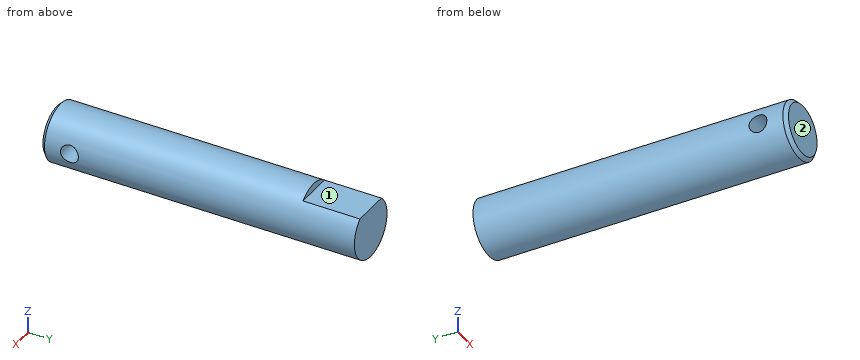
Autodesk Inventor part; units mm, degrees
ref_plane "Work Plane1" through (-4, 0, 0) normal (1, 0, 0) x (0, 1, 0)
ref_plane "XZ Plane" through (0, 0, 0) normal (0, 1, 0) x (-1, 0, 0)
ref_plane "XY Plane" through (0, 0, 0) normal (0, 0, 1) x (1, 0, 0)
sketch "Sketch2" plane through (0, 0, 0) normal (0, 1, 0) x (-1, 0, 0)
  circle A0 centre (0, 0) radius 4
  dimension "d9" = 8
extrude "Extrusion1" add sketch "Sketch2" along normal blind 44
chamfer "Chamfer1" distance 0.5 angle 45 1 edges at (4, 0, 0)
sketch "Sketch3" plane through (0, 44, 0) normal (0, 1, 0) x (1, 0, 0)
  line L0 (0, 0) -> (0, -3) construction
  line L1 (0, -3) -> (-4, -3)
  line L2 (0, -3) -> (4, -3)
  line L3 (4, -3) -> (4, -6)
  line L4 (4, -6) -> (-4, -6)
  line L5 (-4, -6) -> (-4, -3)
  dimension "d15" = 3
  dimension "d16" = 4
  dimension "d17" = 4
  dimension "d18" = 3
extrude "Extrusion2" cut sketch "Sketch3" against normal blind 8
ref_plane "Work Plane1" through (-4, 0, 0) normal (1, 0, 0) x (0, 1, 0)
sketch "Sketch4" plane through (-4, 0, 0) normal (1, 0, 0) x (0, 1, 0)
  line L0 (0.5, 4) -> (0.5, -4) construction
  line L1 (0.5, 0) -> (4, 0) construction
  circle A0 centre (4, 0) radius 1.25
  point P0 (0, 0)
  dimension "d23" = 2.5
  dimension "d24" = 3.5
extrude "Extrusion3" cut sketch "Sketch4" along normal through all
properties part number "reverse gear crankshaft outer rod"
Model file for the job. Use its own axes, mm. Face numbers are marked on the shaded views. A direction names the side the tool comes from. Give positions to 0.01 mm unless a question says otherwise; leave off trailing zeros. Loops run counter-clockwise (first coordinate to the right, second up) from the corner with the lowest first, then second, coordinate; pieces in that order, holes last.
Item 1: Slice it at C-C (y = 4). Write the cut outline in (x, z), plus the area to 3 significant figures.
Check values:
outline: (-3.8, -1.25) arc R4 ccw to (3.8, -1.25) - close; (-3.8, 1.25) - (3.8, 1.25) arc R4 ccw to start
area: 30.6 mm2
Item 2: Drill centre lines: line 1 along Y through (x, z) = (-0.5, 0); line 2 along Z through (x, y) = (0, 4); line 3 along Z through (x, y) = (-3, 3.5). Where is each one in solid material? Low to high.
Check values:
line 1: y = 0 to 2.75, 5.25 to 44
line 2: z = -4 to -1.25, 1.25 to 4
line 3: z = -2.65 to -1.15, 1.15 to 2.65
Item 3: Slice it at D-D (y = 41). Write the cut outline in (x, z).
Check values:
outline: (-2.65, 3) arc R4 ccw (long way) to (2.65, 3) - close
Item 4: Slice it at A-A (z = 0). Write the cut outline in (x, y).
Check values:
outline: (-4, 0.5) - (-3.5, 0) - (3.5, 0) - (4, 0.5) - (4, 2.75) - (-4, 2.75) - close; (-4, 5.25) - (4, 5.25) - (4, 44) - (-4, 44) - close
Item 5: Slice it at B-B (x = 0). Write the cut outline in (y, z), plus the area to 3 significant figures.
Check values:
outline: (0, -3.5) - (0.5, -4) - (44, -4) - (44, 3) - (36, 3) - (36, 4) - (0.5, 4) - (0, 3.5) - close; hole circle Ø2.5 at (4, 0)
area: 339 mm2
Item 6: Drop flat-ended pins along their axis: P1, Ø2, axis at y = 30.5, z = -2, coming from the +X side; P2, Ø1.5, axis at y = 14, z = -1, coming from the +X side; P3, Ø2, axis at x = 2.5, y = 14.5, coming from the -Z side. Give the stop position or say it passes through.
Check values:
P1: stops at x = 3.87
P2: stops at x = 3.99
P3: stops at z = -3.71
Item 7: Which spindle directions (+Z, -Z, +X, -X, +Y, -Y) get a long thin tool onto all of the face, cutting with end or side? Do the marked faces 1 and 2. Say none if no direction does.
Check values:
face 1: +Z, +X, -X, +Y
face 2: +Z, -Z, +X, -X, -Y
